Here's the drawing with two shaded views (mm, measured from the low corner). I have some questions. A direction names the side the tool comes from. Round coordinates to 2 decimals unless told otherwise and drop trailing zeros. Write each loop counter-clockwise with the first axis right and the second up, starting at its lowest first coordinate (ties: lowest second). Pieces come first, ordered by that corner, then holes. Notation, with made-up numbers: (42.5, 82) - (60.5, 82) arc R23 cw to (60.5, 112) - close; hole circle Ø7 at (49, 17.25). An arc over 180 degrees is marked (long way). Return JSON: item names as keys, results as strings. Group by question number.
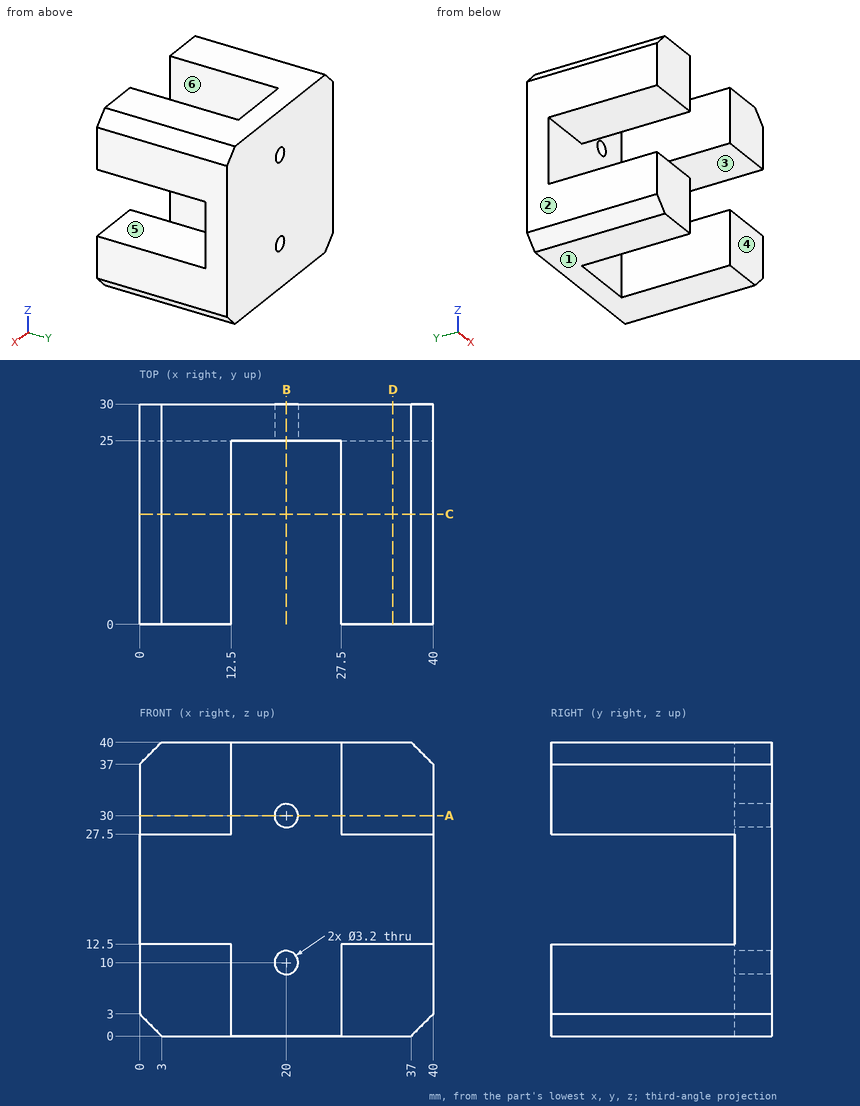
1) Imagine slicing it at A-A (z = 30). Please give me the cut outline in (x, y).
2) Imagine slicing it at B-B (x = 20). Please give me the cut outline in (y, z).
3) If we mould it in two halves opening along Z, with no side actions, what happens to the marked faces 1, 2 and 3? For each: released by +Z, released by -Z, zero draft, split by the parting line, or undercut.
4) Imagine slicing it at D-D (x = 34.5). Please give me the cut outline in (y, z).
5) I need wall thicknesses on line 1 along Z through (x, y) = (20, 28.05); line 2 along X through (y, z) = (20.75, 29.5); line 3 along X through (y, z) = (27.9, 30). Which ranges of each line are inside material? Lowest first, please.
6) For the marked faces 4, 5 and 6, which set-ups out of +Z, -Z, +X, -X, +Y, -Y let a thin tool reach every point of the face, with its end or its side?
7) Will this pin go through, and if not, where does the flat tip stop? pin 1 Ø1.5 at (x, z) = (7, 21.5) entering from -Y.
8) Imagine slicing it at C-C (y = 15). Please give me the cut outline in (x, z), plus the area to 3 significant figures.
Results found:
{
 "1": {"outline": "(0, 0) - (12.5, 0) - (12.5, 25) - (18.4, 25) - (18.4, 30) - (0, 30) - close; (21.6, 25) - (27.5, 25) - (27.5, 0) - (40, 0) - (40, 30) - (21.6, 30) - close"},
 "2": {"outline": "(25, 0) - (30, 0) - (30, 8.4) - (25, 8.4) - close; (25, 11.6) - (30, 11.6) - (30, 28.4) - (25, 28.4) - close; (25, 31.6) - (30, 31.6) - (30, 40) - (25, 40) - close"},
 "3": {"face 1": "released by -Z", "face 2": "zero draft", "face 3": "undercut"},
 "4": {"outline": "(0, 0) - (30, 0) - (30, 40) - (0, 40) - (0, 27.5) - (25, 27.5) - (25, 12.5) - (0, 12.5) - close"},
 "5": {"line 1": "z = 0 to 8.4, 11.6 to 28.4, 31.6 to 40", "line 2": "x = 0 to 12.5, 27.5 to 40", "line 3": "x = 0 to 18.4, 21.6 to 40"},
 "6": {"face 4": "+Z, -Z, +X, -X, -Y", "face 5": "+X, -X, -Y", "face 6": "+Z, -Z, -Y"},
 "7": {"pin 1": "stops at y = 25"},
 "8": {"outline": "(0, 3) - (3, 0) - (12.5, 0) - (12.5, 12.5) - (0, 12.5) - close; (0, 27.5) - (12.5, 27.5) - (12.5, 40) - (3, 40) - (0, 37) - close; (27.5, 0) - (37, 0) - (40, 3) - (40, 12.5) - (27.5, 12.5) - close; (27.5, 27.5) - (40, 27.5) - (40, 37) - (37, 40) - (27.5, 40) - close", "area": "607 mm²"}
}
